The model under review builds one solid part; all positions refer to its coordinate system, in mm. A direction names the side the tool comes from. Give positions to 0.01 mm unless a question says otherwise; leave off trailing zeros. Order: outer loops, then holes, each group sorted by start corner. A loop starts at its lowest first (then second) coordinate and runs counter-clockwise, first axis right, second up. Notation, with made-up numbers: M -34,26.5 L -25,26.5 A18 ccw -25,54.5 Z; hole C -12,70.25 d9. An arc over 180 degrees is marked long. One line per question, with ' | ' between items. Start each with the question number.
1. The part is to be moulded in two halves that separate along Y. For faces 1 (the face through (-2, -80, 9)), 2 (the face through (-2, 23, 19)), 3 (the face through (160, -1, 9)), say which applies: +Y half, -Y half, draft (parallel to the pull), parting line (faces both ways), or undercut.
2. Insertion check: P1, Ø1.5, axis at x = -78.5, z = 20.5, coming from the -Y side; P2, Ø2.5, axis at x = -61, z = 21.5, coming from the +Y side; P3, Ø3, axis at x = 1, y = -66.5, coming from the -Z side. Each pin has a flat end and moves straight along its axis. Give the tip position at first contact, or say it passes through.
3. We need section A-A on z = 9. Count the separate pieces of the cut face and the enclosed holes in it, then the cut area to 3 significant figures.
4. We need section B-B on y = -7.5. Write out the cut boundary in (x, z), then the cut area to 3 significant figures.
5. For faces 4 (the face through (-2, -67, 19)), 5 (the face through (-5, -1, 6)), list the 3-axis set-ups (+Z, -Z, +X, -X, +Y, -Y) from which the entire face can be reached by the end or side of a thin tool; tool diameter is ignored.
6. Wall thickness on L1, parallel to Y at x = 143.75, z = 8.75; L2, parallel to Y at x = 0, z = 7.75; L3, parallel to Y at x = -134.5, z = 6.25: over which ranges is each line inside the solid? List them lowest first.
```python
from build123d import *

# Parameters (mm, degrees)
SKETCH1_W           = 320
SKETCH1_H           = 160
BOSS_EXTRUDE1_DEPTH = 19
SKETCH4_W           = 320
SKETCH4_H           = 1
BOSS_EXTRUDE4_DEPTH = 5
LPATTERN2_COUNT     = 16
LPATTERN2_PITCH     = 10
SKETCH5_W           = 135
SKETCH5_H           = 120
CUT_EXTRUDE1_DEPTH  = 12
SKETCH6_R           = 2
CUT_EXTRUDE2_DEPTH  = 12
SKETCH7_R           = 1.5
BOSS_EXTRUDE5_DEPTH = 4
FILLET2_R           = 1.5


with BuildPart() as part:
    # Sketch1 → Boss-Extrude1 (new body)
    with BuildSketch(Plane.XY):
        Rectangle(SKETCH1_W, SKETCH1_H)
    extrude(amount=BOSS_EXTRUDE1_DEPTH)

    # Sketch4 → Boss-Extrude4 (add)
    with BuildSketch(Plane.XY.offset(19)):
        with Locations((0, 78.3)):
            Rectangle(SKETCH4_W, SKETCH4_H)
    boss_extrude4 = extrude(amount=BOSS_EXTRUDE4_DEPTH)

    # LPattern2: Boss-Extrude4 ×16
    with Locations(*[(0, -i * LPATTERN2_PITCH, 0) for i in range(1, LPATTERN2_COUNT)]):
        add(boss_extrude4)

    # Sketch5 → Cut-Extrude1 (cut)
    with BuildSketch(Plane(origin=(0, 0, 0), x_dir=(-1, 0, 0), z_dir=(0, 0, -1))):
        with Locations((-72.5, 0)):
            Rectangle(SKETCH5_W, SKETCH5_H)
        with Locations((72.5, 0)):
            Rectangle(SKETCH5_W, SKETCH5_H)
    extrude(amount=-CUT_EXTRUDE1_DEPTH, mode=Mode.SUBTRACT)

    # Sketch6 → Cut-Extrude2 (cut)
    with BuildSketch(Plane(origin=(0, 0, 0), x_dir=(-1, 0, 0), z_dir=(0, 0, -1))):
        with Locations((-143.75, 50)):
            Circle(SKETCH6_R)
        with Locations((-143.75, -50)):
            Circle(SKETCH6_R)
        with Locations((0, 66.25)):
            Circle(SKETCH6_R)
        with Locations((143.75, 50)):
            Circle(SKETCH6_R)
        with Locations((143.75, -50)):
            Circle(SKETCH6_R)
        with Locations((0, -66.25)):
            Circle(SKETCH6_R)
    extrude(amount=-CUT_EXTRUDE2_DEPTH, mode=Mode.SUBTRACT)

    # Sketch7 → Boss-Extrude5 (add)
    with BuildSketch(Plane(origin=(0, 0, 0), x_dir=(-1, 0, 0), z_dir=(0, 0, -1))):
        with Locations(Location((-120, 66, 0), (0, 0, 180))):
            Circle(SKETCH7_R)
        with Locations(Location((120, 66, 0), (0, 0, 180))):
            Circle(SKETCH7_R)
        with Locations(Location((120, -66, 0), (0, 0, 180))):
            Circle(SKETCH7_R)
        with Locations(Location((-120, -66, 0), (0, 0, 180))):
            Circle(SKETCH7_R)
    extrude(amount=BOSS_EXTRUDE5_DEPTH)

    # Fillet2
    fillet2_edges = [part.edges().sort_by_distance(p)[0] for p in [
        (118.5, 66, -4),
        (-121.5, 66, -4),
        (-121.5, -66, -4),
        (118.5, -66, -4),
    ]]
    fillet(fillet2_edges, radius=FILLET2_R)


solid = part.part
```
Entries:
1) face 1: -Y half | face 2: undercut | face 3: draft
2) P1: stops at y = -72.2 | P2: stops at y = 78.8 | P3: stops at z = 0
3) separate pieces: 1 | enclosed holes: 8 | area: 18,700 mm^2
4) outline: M -160,0 L -140,0 L -140,12 L -5,12 L -5,0 L 5,0 L 5,12 L 140,12 L 140,0 L 160,0 L 160,19 L -160,19 Z | area: 2,840 mm^2
5) face 4: +Z, +X, -X | face 5: -Z
6) L1: y = -80 to -52, -48 to 48, 52 to 80 | L2: y = -80 to -68.25, -64.25 to 64.25, 68.25 to 80 | L3: y = -80 to -60, 60 to 80
